```python
from build123d import *

# Parameters (mm, degrees)
SALIENTE_EXTRUIR1_DEPTH = 10
CROQUIS2_R              = 20
CORTAR_EXTRUIR1_DEPTH   = 10
CROQUIS3_R              = 20
CORTAR_EXTRUIR2_DEPTH   = 10
CROQUIS5_W              = 60
CROQUIS5_H              = 10
SALIENTE_EXTRUIR3_DEPTH = 55
SALIENTE_EXTRUIR4_DEPTH = 9
CROQUIS8_R              = 20
CORTAR_EXTRUIR3_DEPTH   = 9
CROQUIS9_R              = 20
CORTAR_EXTRUIR4_DEPTH   = 10
CROQUIS11_W             = 94.452906293
CROQUIS11_H             = 104.053500068
CORTAR_EXTRUIR6_DEPTH   = 54
CROQUIS15_W             = 76.60704733
CROQUIS15_H             = 9.910818825
CORTAR_EXTRUIR7_DEPTH   = 76


with BuildPart() as part:
    # Croquis1 → Saliente-Extruir1 (new body)
    with BuildSketch(Plane(origin=(0, 0, 0), x_dir=(1, 0, 0), z_dir=(0, 1, 0))):
        with BuildLine():
            Line((0, 26.904276051), (128.079511341, 26.904276051))
            ThreePointArc((128.079511341, 26.904276051), (154.983787391, 0), (128.079511341, -26.904276051))
            Line((128.079511341, -26.904276051), (0, -26.904276051))
            ThreePointArc((0, -26.904276051), (-26.904276051, 0), (0, 26.904276051))
        make_face()
    extrude(amount=SALIENTE_EXTRUIR1_DEPTH)

    # Croquis2 → Cortar-Extruir1 (cut)
    with BuildSketch(Plane.XZ):
        with Locations(Location((0, 0, 0), (0, 0, 270))):
            Circle(CROQUIS2_R)
    extrude(amount=-CORTAR_EXTRUIR1_DEPTH, mode=Mode.SUBTRACT)

    # Croquis3 → Cortar-Extruir2 (cut)
    with BuildSketch(Plane(origin=(0, 10, 0), x_dir=(1, 0, 0), z_dir=(0, 1, 0))):
        with Locations(Location((127.980340476, 0, 0), (0, 0, 270))):
            Circle(CROQUIS3_R)
    extrude(amount=-CORTAR_EXTRUIR2_DEPTH, mode=Mode.SUBTRACT)

    # Croquis5 → Saliente-Extruir3 (add)
    with BuildSketch(Plane(origin=(0, 0, 0), x_dir=(-1, 0, 0), z_dir=(0, -1, 0))):
        with Locations((-58.558456053, -21.904276051)):
            Rectangle(CROQUIS5_W, CROQUIS5_H)
        with Locations((-58.558456053, 21.904276051)):
            Rectangle(CROQUIS5_W, CROQUIS5_H)
    extrude(amount=SALIENTE_EXTRUIR3_DEPTH)

    # Croquis7 → Saliente-Extruir4 (add)
    with BuildSketch(Plane(origin=(0, -55, 0), x_dir=(-1, 0, 0), z_dir=(0, -1, 0))):
        with BuildLine():
            Line((0, -26.929773303), (-127.980340476, -26.929773303))
            ThreePointArc((-127.980340476, -26.929773303), (-154.910113778, 0), (-127.980340476, 26.929773303))
            Line((-127.980340476, 26.929773303), (0, 26.929773303))
            ThreePointArc((0, 26.929773303), (26.929773303, 0), (0, -26.929773303))
        make_face()
    extrude(amount=SALIENTE_EXTRUIR4_DEPTH)

    # Croquis8 → Cortar-Extruir3 (cut)
    with BuildSketch(Plane(origin=(0, -64, 0), x_dir=(-1, 0, 0), z_dir=(0, -1, 0))):
        with Locations(Location((-129.139989333, 0, 0), (0, 0, 90))):
            Circle(CROQUIS8_R)
    extrude(amount=-CORTAR_EXTRUIR3_DEPTH, mode=Mode.SUBTRACT)

    # Croquis9 → Cortar-Extruir4 (cut)
    with BuildSketch(Plane(origin=(0, -64, 0), x_dir=(-1, 0, 0), z_dir=(0, -1, 0))):
        with Locations(Location((0, 0, 0), (0, 0, 90))):
            Circle(CROQUIS9_R)
    extrude(amount=-CORTAR_EXTRUIR4_DEPTH, mode=Mode.SUBTRACT)

    # Croquis11 → Cortar-Extruir6 (cut)
    with BuildSketch(Plane.XY.offset(26.929773303)):
        with Locations((14.683121645, -22.540401026)):
            Rectangle(CROQUIS11_W, CROQUIS11_H)
    extrude(amount=-CORTAR_EXTRUIR6_DEPTH, mode=Mode.SUBTRACT)

    # Croquis15 → Cortar-Extruir7 (cut)
    with BuildSketch(Plane(origin=(61.909574791, 10, 26.705021593), x_dir=(1, 0, 0), z_dir=(0, 1, 0))):
        with Locations((-38.303523665, -4.955409412)):
            Rectangle(CROQUIS15_W, CROQUIS15_H)
    extrude(amount=-CORTAR_EXTRUIR7_DEPTH, mode=Mode.SUBTRACT)


solid = part.part
```
Work out the finished part from the listing and answer in its coordinate system (mm). A direction names the side the tool comes from. Give positions to 0.01 mm unless a question says otherwise; leave off trailing zeros. Loops run counter-clockwise (first coordinate to the right, second up) from the corner with the lowest first, then second, coordinate; pieces in that order, holes last. Notation, with made-up numbers: (72.25, -0.75) - (92.25, -0.75) arc R19 ccw to (92.25, 6.25) - close; hole circle Ø4 at (46.5, 45). An arc over 180 degrees is marked (long way). Use CSV: the item, a comma, the result in double quotes. Start each with the question number.
(1) Determine the mould class of faces 1 (the face through (80, -23, -26.904)), 2 (the face through (154.904, -59.437, 0.592)), 3 (the face through (148.97, -59.56, 2.6)) for opening direction X: released by +X, released by -X, zero draft, split by the parting line, or undercut.
(2) Find the intervals of material crossed by L1, parallel to Y at x = 119, z = 22; L2, parallel to Z at x = 67, y = -18.5; L3, parallel to X at y = -59, z = 0, in increasing order.
(3) Find section D-D, the plane x = 136.5. Determine the outline of the cut face in (y, z), plus the area to 3 significant figures.
(4) Each of these flat-tipped pins is pushed along its axis until it touches: pin 1 (5 mm diameter, centred on y = -33.5, z = -20, fed in from +X); pin 2 (13.5 mm diameter, centred on x = 73.5, y = -39, fed in from -Z); pin 3 (2 mm diameter, centred on x = 110.5, z = -3, fed in from +Y); pin 4 (1 mm diameter, centred on y = 0.5, z = -10, fed in from +X). Where does it stop, or does it pass through?
(5) Find section A-A, the plane x = 101.5. Determine the outline of the cut face in (y, z).
(6) A tool of negligible diameter and unlimited length cuts with its end or side. For faces 4 (the face through (108.456, 5.07, -4.336)), 5 (the face through (75, -27, -16.904)), 6 (the face through (88.558, -27, -22)), 7 (the face through (108, -55, 0)), from which of +Z, -Z, +X, -X, +Y, -Y can it reach the whole face along a straight path? Write none if from no direction.
(7) Find section C-C, the plane z = 0. Determine the outline of the cut face in (x, y), plus the area to 3 significant figures.
(8) Find section B-B, the plane y = -19. Determine the outline of the cut face in (x, z).
Results found:
1,face 1,"zero draft"
1,face 2,"released by +X"
1,face 3,"undercut"
2,L1,"-64 to -55, 0 to 10"
2,L2,"-26.9 to -16.9, 16.9 to 26.9"
2,L3,"61.91 to 109.14, 149.14 to 154.91"
3,outline,"(-64, -25.55) - (-55, -25.55) - (-55, -18.6) - (-64, -18.6) - close; (-64, 18.6) - (-55, 18.6) - (-55, 25.55) - (-64, 25.55) - close; (0, -25.55) - (10, -25.55) - (10, -18.09) - (0, -18.09) - close; (0, 18.09) - (10, 18.09) - (10, 25.55) - (0, 25.55) - close"
3,area,"274 mm^2"
4,pin 1,"x = 88.56"
4,pin 2,"z = -26.9"
4,pin 3,"through"
4,pin 4,"x = 153.25"
5,outline,"(-64, -26.93) - (-55, -26.93) - (-55, 26.93) - (-64, 26.93) - close; (0, -26.9) - (10, -26.9) - (10, 26.9) - (0, 26.9) - close"
6,face 4,"+Y"
6,face 5,"+X, -X"
6,face 6,"+Z, -Z, +X"
6,face 7,"+X"
7,outline,"(61.91, -64) - (109.14, -64) - (109.14, -55) - (61.91, -55) - close; (61.91, 0) - (107.98, 0) - (107.98, 10) - (61.91, 10) - close; (147.98, 0) - (154.98, 0) - (154.98, 10) - (147.98, 10) - close; (149.14, -64) - (154.91, -64) - (154.91, -55) - (149.14, -55) - close"
7,area,"1,010 mm^2"
8,outline,"(61.91, -26.9) - (88.56, -26.9) - (88.56, -16.9) - (61.91, -16.9) - close; (61.91, 16.9) - (88.56, 16.9) - (88.56, 26.9) - (61.91, 26.9) - close"
